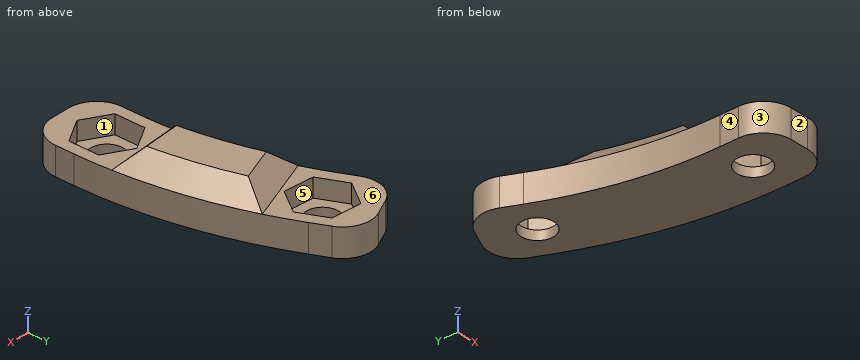
Autodesk Inventor part; units mm, degrees
ref_plane "作業平面1" through (-22.5535, -5, 3) normal (-0.2164396, 0.976296, 0) x (0, 0, -1)
ref_plane "YZ Plane" through (0, 0, 0) normal (1, 0, 0) x (0, 1, 0)
ref_plane "XZ Plane" through (0, 0, 0) normal (0, 1, 0) x (-1, 0, 0)
sketch "スケッチ1" plane through (0, 0, 0) normal (0, 0, 1) x (1, 0, 0)
  arc A0 (46, 0) -> (41.6902, 19.4404) centre (0, 0) ccw construction
  line L0 (0, 0) -> (46, 0) construction
  line L1 (0, 0) -> (46, 0) construction
  line L2 (0, 0) -> (41.6902, 19.4404) construction
  arc A1 (50, 0) -> (45.3154, 21.1309) centre (0, 0) ccw
  arc A2 (42, 0) -> (38.0649, 17.75) centre (0, 0) ccw
  line L3 (42, 0) -> (50, 0)
  line L4 (50, 0) -> (50, -5)
  line L5 (50, -5) -> (42, -5)
  line L6 (42, -5) -> (42, 0)
  line L7 (45.3154, 21.1309) -> (38.0649, 17.75)
  line L8 (38.0649, 17.75) -> (35.9518, 22.2815)
  line L9 (35.9518, 22.2815) -> (43.2023, 25.6625)
  line L10 (43.2023, 25.6625) -> (45.3154, 21.1309)
  dimension "d0" = 46
  dimension "d1" = 0
  dimension "d2" = 25
  dimension "d3" = 4
  dimension "d4" = 4
  dimension "d5" = 8
  dimension "d6" = 5
  dimension "d7" = 5
extrude "押し出し1" add sketch "スケッチ1" along normal blind 3
sketch "スケッチ2" plane through (0, 0, 3) normal (0, 0, 1) x (1, 0, 0)
  arc A0 (46, 0) -> (41.6902, 19.4404) centre (0, 0) ccw construction
  line L0 (0, 0) -> (46, 0) construction
  line L1 (0, 0) -> (46, 0) construction
  line L2 (0, 0) -> (41.6902, 19.4404) construction
  dimension "d10" = 46
  dimension "d11" = 0
  dimension "d12" = 25
hole "穴1" at (41.6902, 19.4404, 3) at (46, 0, 3) direction (0, 0, -1) diameter 3.5 end through all
sketch "スケッチ3" plane through (0, 0, 3) normal (0, 0, 1) x (1, 0, 0)
  circle A0 centre (46, 0) radius 1.75
  line L0 (46, 3.2332) -> (48.8, 1.6166)
  line L1 (48.8, 1.6166) -> (48.8, -1.6166)
  line L2 (48.8, -1.6166) -> (46, -3.2332)
  line L3 (46, -3.2332) -> (43.2, -1.6166)
  line L4 (43.2, -1.6166) -> (43.2, 1.6166)
  line L5 (43.2, 1.6166) -> (46, 3.2332)
  point P0 (0, 0)
  dimension "d20" = 5.6
extrude "押し出し2" cut sketch "スケッチ3" against normal blind 2
pattern_circular "円形状パターン1" count 2 over 25 about axis through (0, 0, -10) along (0, 0, 1) of "押し出し2"
ref_plane "作業平面1" through (-22.5535, -5, 3) normal (-0.2164396, 0.976296, 0) x (0, 0, -1)
sketch "スケッチ4" plane through (-22.5535, -5, 3) normal (-0.2164396, 0.976296, 0) x (0, 0, -1)
  line L0 (3, -73.1011) -> (0, -73.1011)
  line L1 (0, -65.1011) -> (3, -65.1011)
  line L2 (0, -65.1011) -> (0, -64.1056)
  line L3 (0, -73.1011) -> (0, -65.1011)
  line L4 (0, -65.1011) -> (-2, -67.1011)
  line L5 (-2, -67.1011) -> (-2, -71.1011)
  line L6 (0, -71.9159) -> (0, -73.1011)
  line L7 (-2, -71.1011) -> (0, -73.1011)
  line L8 (4, -23.1011) -> (-3, -23.1011)
  point P0 (3, -23.1011)
  dimension "d26" = 45
  dimension "d27" = 45
  dimension "d28" = 2
revolve "回転1" add sketch "スケッチ4" angle 16 mid plane about axis through (0, 0, -10) along (0, 0, 1)
chamfer "面取り1" distance 2 angle 45 2 edges at (43.0869, 16.1095, 5) (45.8582, 3.6091, 5)
fillet "フィレット1" radius 3 4 edges at (43.2023, 25.6625, 1.5) (35.9518, 22.2815, 1.5) (50, -5, 1.5) (42, -5, 1.5)
equation "\"d4\" = d3"
equation "\"d6\" = d7"
equation "\"d27\" = d26"
properties part number "3D_frame-connect-base2-2_3D プリント"
The listing builds one solid part. Answer for the finished solid, in the listing's coordinates (mm). Face numbers are marked on the shaded views. A direction names the side the tool comes from. Give positions to 0.01 mm unless a question says otherwise; leave off trailing zeros. Loops run counter-clockwise (first coordinate to the right, second up) from the corner with the lowest first, then second, coordinate; pieces in that order, holes last. Notation, with made-up numbers: (87.25, 36) - (109.25, 36) arc R14 ccw to (109.25, 40) - close; hole circle Ø9 at (56.25, 51). An arc over 180 degrees is marked (long way). Answer as a JSON object with one key per item and string values.
1. Flat-ended cylindrical pins translate along their axes: pin 1 Ø6.5 at (x, y) = (41, 19.5) entering from +Z; pin 2 Ø4.5 at (x, y) = (46, 0) entering from +Z; pin 3 Ø0.6 at (y, z) = (-0.5, 1.5) entering from -X. Find the tip coordinate at first contact, or state that the pin passes through.
Determined:
{"pin 1": "z = 3", "pin 2": "z = 1", "pin 3": "x = 42"}
2. A cutting plane is placed at B-B (y = -1). Write down the section's boundary in (x, z), then the cut area to 3 significant figures.
Determined:
{"outline": "(42, 0) - (44.56, 0) - (44.56, 1) - (43.2, 1) - (43.2, 3) - (42, 3) - close; (47.44, 0) - (50, 0) - (50, 3) - (48.8, 3) - (48.8, 1) - (47.44, 1) - close", "area": "9.93 mm²"}
3. Find the intervals of material crossed by L1, parallel to X at y = 0, z = 0.45; L2, parallel to Y at x = 44, z = 1.6; L3, parallel to X at y = -0.75, z = 2.5, in increasing order. Write a range as [from, to].
Determined:
{"L1": "[42, 44.25], [47.75, 50]", "L2": "[-4.83, -2.08], [2.08, 17.86], [21.11, 23.66]", "L3": "[42, 43.2], [48.8, 50]"}
4. For a pull along X with two mould halves and no side action, classify the marked faces 1, 2 and 3 as pulls with the +X half, pulls with the -X half, needs draft (parallel to the pull), parting line crosses it, or undercut.
Determined:
{"face 1": "undercut", "face 2": "needs draft", "face 3": "pulls with the -X half"}
5. For the marked faces 4, 5 and 6, determine the directions among +Z, -Z, +X, -X, +Y, -Y from which every point of the face is accessible in a straight line to the end or side of a thin tool.
Determined:
{"face 4": "+Z, -Z, -X, -Y", "face 5": "+Z", "face 6": "+Z, -X, +Y"}
6. A cutting plane is placed at A-A (z = 1.35). Write down the section's boundary in (x, y), then the cut area to 3 significant figures.
Determined:
{"outline": "(37.22, 19.56) - (38.06, 17.75) arc R42 cw to (42, 0) - (42, -2) arc R3 ccw to (45, -5) - (47, -5) arc R3 ccw to (50, -2) - (50, 0) arc R50 ccw to (45.32, 21.13) - (44.47, 22.94) arc R3 ccw to (40.48, 24.39) - (38.67, 23.55) arc R3 ccw to start; hole (38.47, 19.72) - (39.84, 16.79) - (43.06, 16.51) - (44.91, 19.16) - (43.54, 22.09) - (40.32, 22.37) - close; hole (43.2, -1.62) - (46, -3.23) - (48.8, -1.62) - (48.8, 1.62) - (46, 3.23) - (43.2, 1.62) - close", "area": "179 mm²"}
